Could you check a few things on this drawing? It's one solid part, dimensions in mm from its lowest x, y, z. A direction names the side the tool comes from. Give positions to 0.01 mm unless a question says otherwise; leave off trailing zeros. Order: outer loops, then holes, each group sorted by start corner. A loop starts at its lowest first (then second) coordinate and runs counter-clockwise, first axis right, second up.
(1) If I drill on probe 1 along X at (y, z) = (12.5, 2.25); probe 2 along X at (y, z) = (1.15, 12.7), over which ranges is the centre line in solid material (lowest first)?
(2) Imagine slicing it at A-A, the plane z = 12.7. Write out the boundary of the cut face in (x, y).
(3) Will these pins go through, and if not, where does the flat tip stop? pin 1 (12 mm diameter, centred on y = 23, z = 10, fed in from +X); pin 2 (7.5 mm diameter, centred on x = 22, z = 10, fed in from +Y); pin 3 (4.5 mm diameter, centred on y = 15.875, z = 12.7, fed in from +X); pin 4 (4 mm diameter, centred on y = 27.5, z = 5, fed in from -X).
(4) Imagine slicing it at C-C, the plane x = 27. Write out the boundary of the cut face in (y, z).
(5) On a 3-axis mill with a long thin cutter (end or side, diameter ignored), from which of +Z, -Z, +X, -X, +Y, -Y can I reach the whole of each face in a straight line? I mean the marked faces 1 and 2. Say none if no direction works.
(6) Imagine slicing it at B-B, the plane z = 6. Write out the boundary of the cut face in (x, y).
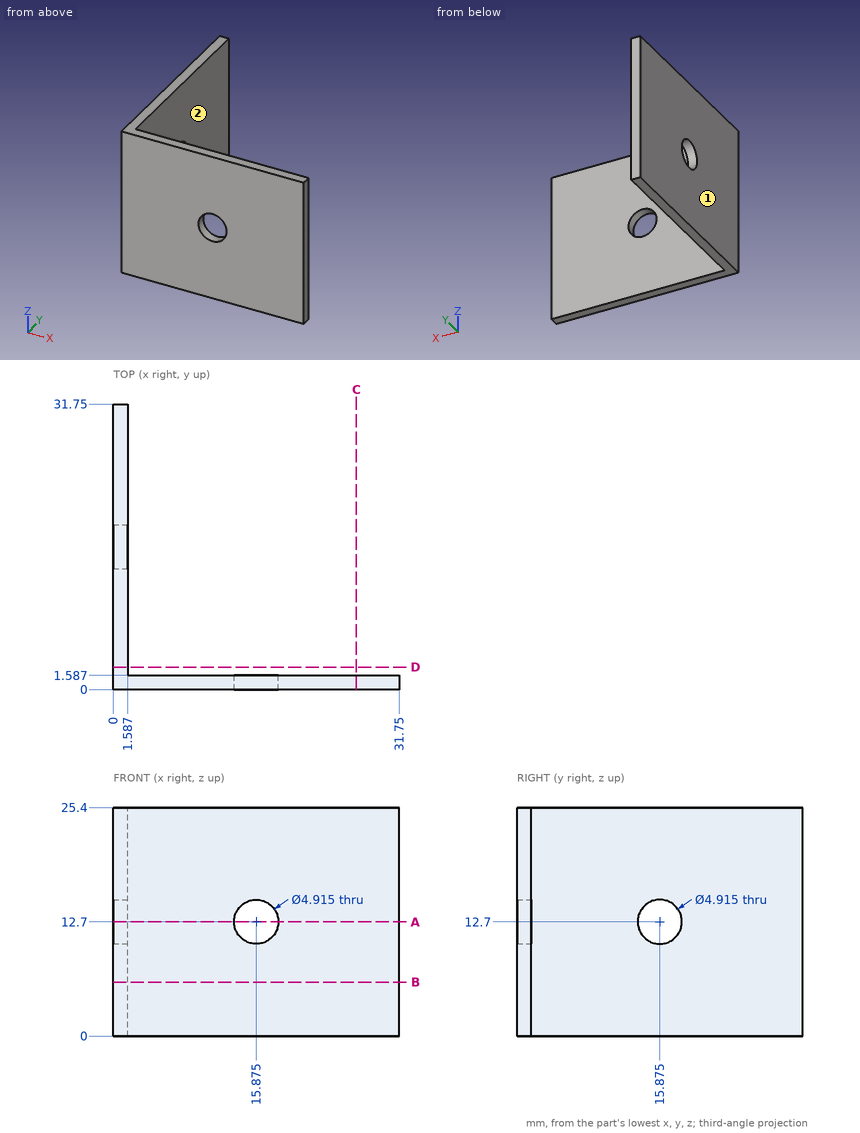
Answer block:
1. probe 1: x = 0 to 1.59
1. probe 2: x = 0 to 13.42, 18.33 to 31.75
2. outline: (0, 0) - (13.42, 0) - (13.42, 1.59) - (1.59, 1.59) - (1.59, 13.42) - (0, 13.42) - close; (0, 18.33) - (1.59, 18.33) - (1.59, 31.75) - (0, 31.75) - close; (18.33, 0) - (31.75, 0) - (31.75, 1.59) - (18.33, 1.59) - close
3. pin 1: stops at x = 1.59
3. pin 2: stops at y = 1.59
3. pin 3: passes through
3. pin 4: stops at x = 0
4. outline: (0, 0) - (1.59, 0) - (1.59, 25.4) - (0, 25.4) - close
5. face 1: +Z, -Z, -X, +Y, -Y
5. face 2: +Z, -Z, +X, +Y
6. outline: (0, 0) - (31.75, 0) - (31.75, 1.59) - (1.59, 1.59) - (1.59, 31.75) - (0, 31.75) - close
